Geometry check sheet. Reference: the model listing, model coordinates, mm. A direction names the side the tool comes from. Round coordinates to 2 decimals unless told otherwise and drop trailing zeros. Loops run counter-clockwise (first coordinate to the right, second up) from the corner with the lowest first, then second, coordinate; pieces in that order, holes last. Notation, with made-up numbers: M 42.5,-2 L 99.5,-2 A11 cw 99.5,6 Z; hole C 50,9.5 d9. An arc over 180 degrees is marked long. Write item = value, one per line.
from build123d import *

# Parameters (mm, degrees)
F1_W          = 75
F1_H          = 10
F2_ANGLE_BACK = 15
F2_ANGLE      = 30
F3_DEPTH      = 1
F5_DEPTH      = 5


with BuildPart() as f2:
    # F1 (on Right) → F2 (revolve)
    with BuildSketch(Plane.YZ, mode=Mode.PRIVATE) as f2_sk:
        with Locations((37.5, 5)):
            Rectangle(F1_W, F1_H)
    revolve(f2_sk.sketch.rotate(Axis((0, -138, 25.0724516809), (0, 0, 1)), -F2_ANGLE_BACK), axis=Axis((0, -138, 25.0724516809), (0, 0, 1)), revolution_arc=F2_ANGLE)

    # F0 (on Top) → F3 (cut)
    with BuildSketch(Plane.XY):
        with BuildLine():
            Line((-21.1415446532, 99.0594758487), (-12.4259198532, -0.5605714658))
            ThreePointArc((-12.4259198532, -0.5605714658), (-12.0274924992, -0.5251316633), (-11.6289640948, -0.4908468716))
            Line((-11.6289640948, -0.4908468716), (-20.3445888947, 99.1292004429))
            Line((-20.3445888947, 99.1292004429), (-21.1415446532, 99.0594758487))
        make_face()
        with BuildLine():
            Line((-16.5406704722, 99.4248643684), (-9.7584498559, -0.3454590055))
            ThreePointArc((-9.7584498559, -0.3454590055), (-9.359410193, -0.3177519037), (-8.9602918959, -0.2912015551))
            Line((-8.9602918959, -0.2912015551), (-15.7425125122, 99.4791218187))
            Line((-15.7425125122, 99.4791218187), (-16.5406704722, 99.4248643684))
        make_face()
        with BuildLine():
            Line((-11.9335760215, 99.7009671064), (-7.0873101046, -0.1821127884))
            ThreePointArc((-7.0873101046, -0.1821127884), (-6.6878081953, -0.1621488069), (-6.2882500977, -0.1433428858))
            Line((-6.2882500977, -0.1433428858), (-11.1345160146, 99.739737009))
            Line((-11.1345160146, 99.739737009), (-11.9335760215, 99.7009671064))
        make_face()
        with BuildLine():
            Line((-7.3219938409, 99.8876802321), (-4.4135051058, -0.0705942423))
            ThreePointArc((-4.4135051058, -0.0705942423), (-4.0136911865, -0.0583808887), (-3.6138435458, -0.0473264673))
            Line((-3.6138435458, -0.0473264673), (-6.5223322808, 99.9109480071))
            Line((-6.5223322808, 99.9109480071), (-7.3219938409, 99.8876802321))
        make_face()
        with BuildLine():
            Line((-2.7076581579, 99.98493353), (-1.7380403683, -0.0109453048))
            ThreePointArc((-1.7380403683, -0.0109453048), (-1.3380647927, -0.006487172), (-0.9380779751, -0.0031884074))
            Line((-0.9380779751, -0.0031884074), (-1.9076957647, 99.9926904274))
            Line((-1.9076957647, 99.9926904274), (-2.7076581579, 99.98493353))
        make_face()
        with BuildLine():
            ThreePointArc((0.9380779751, -0.0031884074), (1.3380647927, -0.006487172), (1.7380403683, -0.0109453048))
            Line((1.7380403683, -0.0109453048), (2.7076581579, 99.98493353))
            Line((2.7076581579, 99.98493353), (1.9076957647, 99.9926904274))
            Line((1.9076957647, 99.9926904274), (0.9380779751, -0.0031884074))
        make_face()
        with BuildLine():
            ThreePointArc((3.6138435458, -0.0473264673), (4.0136911865, -0.0583808887), (4.4135051058, -0.0705942423))
            Line((4.4135051058, -0.0705942423), (7.3219938409, 99.8876802321))
            Line((7.3219938409, 99.8876802321), (6.5223322808, 99.9109480071))
            Line((6.5223322808, 99.9109480071), (3.6138435458, -0.0473264673))
        make_face()
        with BuildLine():
            ThreePointArc((6.2882500977, -0.1433428858), (6.6878081953, -0.1621488069), (7.0873101046, -0.1821127884))
            Line((7.0873101046, -0.1821127884), (11.9335760215, 99.7009671064))
            Line((11.9335760215, 99.7009671064), (11.1345160146, 99.739737009))
            Line((11.1345160146, 99.739737009), (6.2882500977, -0.1433428858))
        make_face()
        with BuildLine():
            ThreePointArc((8.9602918959, -0.2912015551), (9.359410193, -0.3177519037), (9.7584498559, -0.3454590055))
            Line((9.7584498559, -0.3454590055), (16.5406704722, 99.4248643684))
            Line((16.5406704722, 99.4248643684), (15.7425125122, 99.4791218187))
            Line((15.7425125122, 99.4791218187), (8.9602918959, -0.2912015551))
        make_face()
        with BuildLine():
            ThreePointArc((12.0274924992, -0.5251316633), (12.2267190167, -0.5427072066), (12.4259198532, -0.5605714658))
            Line((12.4259198532, -0.5605714658), (21.1415446532, 99.0594758487))
            Line((21.1415446532, 99.0594758487), (20.3445888947, 99.1292004429))
            Line((20.3445888947, 99.1292004429), (11.6289640948, -0.4908468716))
            ThreePointArc((11.6289640948, -0.4908468716), (11.828240719, -0.5078448729), (12.0274924992, -0.5251316633))
        make_face()
    extrude(amount=F3_DEPTH, mode=Mode.SUBTRACT)

    # F4 (on face) → F5 (cut)
    with BuildSketch(Plane.XY.offset(10)):
        with BuildLine():
            ThreePointArc((42.0580948292, 18.962946772), (128.9199177973, -39.0762677861), (162.5, -138))
            ThreePointArc((162.5, -138), (-98.9237322139, -266.9199177973), (-42.0580948292, 18.962946772))
            Line((-42.0580948292, 18.962946772), (-45.345096702, 31.2302047658))
            ThreePointArc((-45.345096702, 31.2302047658), (-106.6550023623, -276.995505219), (175.2, -138))
            ThreePointArc((175.2, -138), (138.995505219, -31.3449976377), (45.345096702, 31.2302047658))
            Line((45.345096702, 31.2302047658), (42.0580948292, 18.962946772))
        make_face()
        with BuildLine():
            ThreePointArc((-42.0580948292, 18.962946772), (0, 24.5), (42.0580948292, 18.962946772))
            Line((42.0580948292, 18.962946772), (45.345096702, 31.2302047658))
            ThreePointArc((45.345096702, 31.2302047658), (0, 37.2), (-45.345096702, 31.2302047658))
            Line((-45.345096702, 31.2302047658), (-42.0580948292, 18.962946772))
        make_face()
    extrude(amount=-F5_DEPTH, mode=Mode.SUBTRACT)


solid = f2.part
(1) Sectioned sample at D-D on x = 17. Record the cut outline in (y, z), then the cut area to 3 significant figures.
Result set:
outline = M -1.05,0 L 51.72,0 L 51.72,1 L 60.9,1 L 60.9,0 L 74.32,0 L 74.32,10 L 36.37,10 L 36.37,5 L 23.61,5 L 23.61,10 L -1.05,10 Z
area = 681 mm2
(2) Sectioned sample at B-B on x = 39. Record the cut outline in (y, z), then the cut area to 3 significant figures.
Result set:
outline = M 7.55,0 L 71.4,0 L 71.4,10 L 32.8,10 L 32.8,5 L 19.75,5 L 19.75,10 L 7.55,10 Z
area = 573 mm2
(3) Sectioned sample at C-C on x = -34. Record the cut outline in (y, z), then the cut area to 3 significant figures.
Result set:
outline = M -4.25,0 L 72.27,0 L 72.27,10 L 33.87,10 L 33.87,5 L 20.9,5 L 20.9,10 L -4.25,10 Z
area = 700 mm2
(4) Tool access check on faces 4 (the flat face through (-12.337, 37.592, 0.493)), 5 (the flat face through (-1, 28, 5)), 6 (the flat face through (31, 35, 0)). Record the directions out of +Z, -Z, +X, -X, +Y, -Y that give a thin tool (end or side, any length) a straight path to the whole face; none if there is none.
Result set:
face_4 = -Z
face_5 = +Z
face_6 = -Z, +X, -X, +Y, -Y
(5) Sectioned sample at A-A on z = 7. Record the cut outline in (x, y).
Result set:
outline = M -55.13,67.74 L -45.35,31.23 A175.2 cw 45.35,31.23 L 55.13,67.74 A213 ccw Z; M -42.06,18.96 L -35.72,-4.7 A138 cw 35.72,-4.7 L 42.06,18.96 A162.5 ccw Z
(6) Release check for a two-part mould opening along X. For faces 1 (the flat face through (-4, 41, 0)), 2 (the flat face through (-45.287, 31.013, 3.959)), 3 (the flat face through (5, 38, 1)) record: released by +X, released by -X, zero draft, split by the parting line, or undercut.
Result set:
face_1 = zero draft
face_2 = released by -X
face_3 = undercut
(7) Material ranges on line 1 along Y through (x, z) = (-5, 4.25); line 2 along Z through (x, y) = (-10.5, 71); line 3 along Z through (x, y) = (12.5, 35), recorded low to high. Write a range as from..to.
Result set:
line_1 = -0.09..74.94
line_2 = 1..10
line_3 = 0..5
(8) Depth check by flat-ended pin: pin 1 Ø3 at (x, z) = (8.5, 5.5) entering from -Y; pin 2 Ø2 at (y, z) = (37, 1.5) entering from +X; pin 3 Ø2 at (y, z) = (41.5, 7) entering from +X. Enter the tip coordinate at first touch or a pass-through.
Result set:
pin_1 = -0.36
pin_2 = 47.16
pin_3 = 48.36
